Input: part model. Units: mm. Frame: model coordinates. Round coordinates to 2 decimals unless told otherwise and drop trailing zeros. Loops run counter-clockwise (first coordinate to the right, second up) from the corner with the lowest first, then second, coordinate; pieces in that order, holes last. Notation, with made-up numbers: (70, 6) -> (76, 6) arc R5 cw to (76, 11) -> close; hole circle Ø8 at (-12.75, 38.25). An arc over 180 degrees is marked (long way). Answer as a JSON object with one key per item and string values.
```python
from build123d import *


with BuildPart() as part:
    # Sketch1 → Revolve1 (revolve)
    with BuildSketch(Plane.XY):
        with BuildLine():
            Line((-26, 0), (26, 0))
            Line((26, 0), (26, -10))
            ThreePointArc((26, -10), (25.5, -10.133974596), (25, -10))
            Line((25, -10), (25, -5))
            Line((25, -5), (-25, -5))
            Line((-25, -5), (-25, -10))
            ThreePointArc((-25, -10), (-25.5, -10.133974596), (-26, -10))
            Line((-26, -10), (-26, 0))
        make_face()
    revolve(axis=Axis((-26, 0, 0), (1, 0, 0)))


solid = part.part
```
1) Contact query for flat-ended pins moving along their axis: P1, Ø8, axis at x = -13, z = -1, coming from the +Y side; P2, Ø5, axis at x = -20.5, z = 4.5, coming from the +Y side; P3, Ø3, axis at x = 16, y = 5, coming from the -Z side. Output: stop coordinate, or through.
Output:
{"P1": "stops at y = 5", "P2": "stops at y = 4.58", "P3": "stops at z = -3.57"}
2) Section C-C, the plane x = 23.5. Output: boundary loops of the cut face in (y, z), plus the area to 3 significant figures.
Output:
{"outline": "circle Ø10 at (0, 0)", "area": "78.5 mm^2"}
3) Draft query along X for faces 1 (the face through (25, -2, -5)), 2 (the face through (-26, 0, 0)), 3 (the face through (26, 0, 0)). Return one class per face: +X half, -X half, draft (parallel to the pull), parting line (faces both ways), or undercut.
Output:
{"face 1": "undercut", "face 2": "-X half", "face 3": "+X half"}
4) Ray query, probe 1 along X at (y, z) = (5.75, -3.5); probe 2 along Z at (x, y) = (-14, 0); probe 3 along Y at (x, z) = (9.5, 0.5). Return the intervals inside material, ascending.
Output:
{"probe 1": "x = -26 to -25, 25 to 26", "probe 2": "z = -5 to 5", "probe 3": "y = -4.97 to 4.97"}
5) Section A-A, the plane y = 0. Output: boundary loops of the cut face in (x, z), plus the area to 3 significant figures.
Output:
{"outline": "(-26, -10) arc R1 ccw to (-25, -10) -> (-25, -5) -> (25, -5) -> (25, -10) arc R1 ccw to (26, -10) -> (26, 10) arc R1 ccw to (25, 10) -> (25, 5) -> (-25, 5) -> (-25, 10) arc R1 ccw to (-26, 10) -> close", "area": "540 mm^2"}
